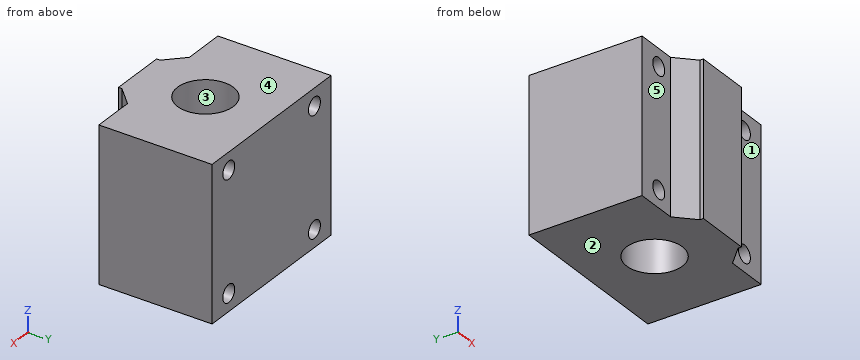
from build123d import *

# Parameters (mm, degrees)
SKETCH_1_R          = 8
EXTRUDE_1_DEPTH     = 44
SKETCH_2_R          = 2.5
CUT_EXTRUDE_1_DEPTH = 64.586555183


with BuildPart() as part:
    # 草图1 → 凸台-拉伸1 (new body)
    with BuildSketch(Plane.XY):
        Polygon((8, 0), (-8, 0), (-8, 1), (-13, 6), (-25, 6), (-25, 38.5), (25, 38.5), (25, 6), (13, 6), (8, 1), align=None)
        with Locations((0, 19.5)):
            Circle(SKETCH_1_R, mode=Mode.SUBTRACT)
    extrude(amount=EXTRUDE_1_DEPTH)

    # 草图2 → 切除-拉伸1 (cut, through all)
    with BuildSketch(Plane(origin=(0, 38.5, 0), x_dir=(1, 0, 0), z_dir=(0, 1, 0))):
        with Locations(Location((-18, -5, 0), (0, 0, 270))):
            Circle(SKETCH_2_R)
        with Locations(Location((18, -5, 0), (0, 0, 270))):
            Circle(SKETCH_2_R)
        with Locations(Location((18, -39, 0), (0, 0, 270))):
            Circle(SKETCH_2_R)
        with Locations(Location((-18, -39, 0), (0, 0, 270))):
            Circle(SKETCH_2_R)
    extrude(amount=-CUT_EXTRUDE_1_DEPTH, mode=Mode.SUBTRACT)


solid = part.part
Input: part model. Units: mm. Frame: model coordinates. Face numbers are marked on the shaded views. A direction names the side the tool comes from. Coordinates: 2 decimals unless noted, no trailing zeros. Loops run counter-clockwise (first coordinate to the right, second up) from the corner with the lowest first, then second, coordinate; pieces in that order, holes last. Notation, with made-up numbers: (9, -31) -> (37, -31) arc R14 ccw to (37, -7) -> close; hole circle Ø2 at (-18.75, -30). An arc over 180 degrees is marked (long way). Write each question's results on one line, items separated by ' | '. Start each with the question number.
Q1. Reachability of the marked faces 4 and 5 from +Z, -Z, +X, -X, +Y, -Y: full face, straight path, thin tool, end or side. Return the list, or none.
Q2. Pin query (flat end, axial travel): pin 1 (4.5 mm diameter, centred on x = -18, z = 5, fed in from -Y); pin 2 (6 mm diameter, centred on x = -18, z = 39, fed in from -Y); pin 3 (13 mm diameter, centred on x = 18.5, z = 13, fed in from -Y); pin 4 (1.5 mm diameter, centred on y = 4.5, z = 19, fed in from +X). Return the tip coordinate at first contact, or that it passes through.
Q3. Ray query, line 1 (X direction, y = 9, z = 37); line 2 (X direction, y = 25, z = 5); line 3 (X direction, y = 13, z = 5). Return the intervals inside material, ascending. Write a range as from..to.
Q4. Section B-B, the plane z = 5. Return the cut outline in (x, y).
Q5. Section A-A, the plane x = -18. Return the cut outline in (y, z).
Q6. Section D-D, the plane y = 7. Return the cut outline in (x, z), plus the area to 3 significant figures.
Q7. Pull-direction query (Y, two-part tool) for the marked faces 1, 2 and 3; classes: released by +Y, released by -Y, zero draft, split by the parting line, or undercut.
Q8. Section C-C, the plane y = 23. Return the cut outline in (x, z).
Found:
1) face 4: +Z, +X, -X, +Y, -Y | face 5: +Z, -Z, -X, -Y
2) pin 1: through | pin 2: y = 6 | pin 3: y = 5 | pin 4: x = 12.25
3) line 1: -25..-19.5, -16.5..16.5, 19.5..25 | line 2: -25..-20.5, -15.5..-5.81, 5.81..15.5, 20.5..25 | line 3: -25..-20.5, -15.5..-4.66, 4.66..15.5, 20.5..25
4) outline: (-25, 6) -> (-20.5, 6) -> (-20.5, 38.5) -> (-25, 38.5) -> close; (-15.5, 6) -> (-13, 6) -> (-8, 1) -> (-8, 0) -> (8, 0) -> (8, 1) -> (13, 6) -> (15.5, 6) -> (15.5, 38.5) -> (-15.5, 38.5) -> close; (20.5, 6) -> (25, 6) -> (25, 38.5) -> (20.5, 38.5) -> close; hole circle Ø16 at (0, 19.5)
5) outline: (6, 0) -> (38.5, 0) -> (38.5, 2.5) -> (6, 2.5) -> close; (6, 7.5) -> (38.5, 7.5) -> (38.5, 36.5) -> (6, 36.5) -> close; (6, 41.5) -> (38.5, 41.5) -> (38.5, 44) -> (6, 44) -> close
6) outline: (-25, 0) -> (25, 0) -> (25, 44) -> (-25, 44) -> close; hole circle Ø5 at (-18, 5); hole circle Ø5 at (-18, 39); hole circle Ø5 at (18, 5); hole circle Ø5 at (18, 39) | area: 2,120 mm2
7) face 1: released by -Y | face 2: zero draft | face 3: undercut
8) outline: (-25, 0) -> (-7.19, 0) -> (-7.19, 44) -> (-25, 44) -> close; (7.19, 0) -> (25, 0) -> (25, 44) -> (7.19, 44) -> close; hole circle Ø5 at (-18, 5); hole circle Ø5 at (-18, 39); hole circle Ø5 at (18, 5); hole circle Ø5 at (18, 39)
